Build history of the part. All positions in model axes, mm. Round coordinates to 2 decimals unless told otherwise and drop trailing zeros. Order: outer loops, then holes, each group sorted by start corner. A loop starts at its lowest first (then second) coordinate and runs counter-clockwise, first axis right, second up. Notation, with made-up numbers: (74, 58) -> (81, 58) arc R17 ccw to (81, 89) -> close; hole circle Ø3 at (14.5, 63). An arc over 180 degrees is marked (long way). Answer as a JSON object with one key per item and string values.
from build123d import *

# Parameters (mm, degrees)
SKETCH1_R           = 4.09575
SKETCH1_R_2         = 1.651
BOSS_EXTRUDE1_DEPTH = 6.35
SKETCH3_R           = 1.5875
CUT_EXTRUDE1_DEPTH  = 6.35
CUT_EXTRUDE2_DEPTH  = 6.35
SKETCH7_R           = 4.9784
CUT_EXTRUDE3_DEPTH  = 131.317526076
FILLET1_R           = 6.35
SKETCH8_W           = 50.8
SKETCH8_H           = 38.1
CUT_EXTRUDE4_DEPTH  = 50.8
CUT_EXTRUDE5_DEPTH  = 19.304
FILLET6_R           = 6.35
FILLET8_R           = 19.05
SKETCH10_R          = 1.5875
CUT_EXTRUDE6_DEPTH  = 6.35
SKETCH11_R          = 1.5875
CUT_EXTRUDE7_DEPTH  = 6.35
BOSS_EXTRUDE2_DEPTH = 6.35
FILLET9_R           = 24.13


with BuildPart() as part:
    # Sketch1 → Boss-Extrude1 (new body)
    with BuildSketch(Plane.XY):
        with BuildLine():
            Line((0, 0), (107.95, 0))
            Line((107.95, 0), (100.9362606, 26.175631792))
            Line((100.9362606, 26.175631792), (96.600438298, 42.357140917))
            ThreePointArc((96.600438298, 42.357140917), (108.063690957, 58.995863967), (92.935889192, 72.39))
            Line((92.935889192, 72.39), (0, 38.1))
            Line((0, 38.1), (0, 25.4))
            Line((0, 25.4), (-7.62, 25.4))
            Line((-7.62, 25.4), (-7.62, 12.7))
            Line((-7.62, 12.7), (0, 12.7))
            Line((0, 12.7), (0, 0))
        make_face()
        with Locations((92.935889192, 57.15)):
            Circle(SKETCH1_R, mode=Mode.SUBTRACT)
        with Locations((25.817011896, 25.817011896)):
            Circle(SKETCH1_R_2, mode=Mode.SUBTRACT)
        with Locations((25.817011896, 12.282988104)):
            Circle(SKETCH1_R_2, mode=Mode.SUBTRACT)
        with Locations((12.282988104, 12.282988104)):
            Circle(SKETCH1_R_2, mode=Mode.SUBTRACT)
        with Locations((12.282988104, 25.817011896)):
            Circle(SKETCH1_R_2, mode=Mode.SUBTRACT)
    extrude(amount=BOSS_EXTRUDE1_DEPTH)

    # Sketch3 → Cut-Extrude1 (cut)
    with BuildSketch(Plane.ZY):
        with Locations(Location((3.175, 31.75, 0), (0, 0, 270))):
            Circle(SKETCH3_R)
        with Locations(Location((3.175, 6.35, 0), (0, 0, 270))):
            Circle(SKETCH3_R)
    extrude(amount=-CUT_EXTRUDE1_DEPTH, mode=Mode.SUBTRACT)

    # Sketch6 → Cut-Extrude2 (cut)
    with BuildSketch(Plane.XY.offset(6.35)):
        with BuildLine():
            Line((50.8, 0), (76.2, 0))
            ThreePointArc((76.2, 0), (63.5, 12.7), (50.8, 0))
        make_face()
    extrude(amount=-CUT_EXTRUDE2_DEPTH, mode=Mode.SUBTRACT)

    # Sketch7 → Cut-Extrude3 (cut, through all)
    with BuildSketch(Plane.XY.offset(6.35)):
        with Locations((19.05, 19.05)):
            Circle(SKETCH7_R)
    extrude(amount=-CUT_EXTRUDE3_DEPTH, mode=Mode.SUBTRACT)

    # Fillet1
    fillet1_edges = [part.edges().sort_by_distance(p)[0] for p in [
        (96.600438298, 42.357140917, 3.175),
    ]]
    fillet(fillet1_edges, radius=FILLET1_R)

    # Sketch8 → Cut-Extrude4 (cut)
    with BuildSketch(Plane.XY.offset(6.35)):
        with Locations((25.4, 57.15)):
            Rectangle(SKETCH8_W, SKETCH8_H)
    extrude(amount=-CUT_EXTRUDE4_DEPTH, mode=Mode.SUBTRACT)

    # Sketch9 → Cut-Extrude5 (cut)
    with BuildSketch(Plane.XY.offset(6.35)):
        Polygon((50.8, 56.84337261), (50.8, 40.64), (57.15, 40.64), (57.15, 59.186294187), align=None)
    extrude(amount=-CUT_EXTRUDE5_DEPTH, mode=Mode.SUBTRACT)

    # Fillet6
    fillet6_edges = [part.edges().sort_by_distance(p)[0] for p in [
        (57.15, 40.64, 3.175),
    ]]
    fillet(fillet6_edges, radius=FILLET6_R - 0.0001)  # a hair under: the kernel refuses the full size

    # Fillet8
    fillet8_edges = [part.edges().sort_by_distance(p)[0] for p in [
        (50.8, 0, 3.175),
    ]]
    fillet(fillet8_edges, radius=FILLET8_R)

    # Sketch10 → Cut-Extrude6 (cut)
    with BuildSketch(Plane.XZ):
        with Locations(Location((97.79, 3.175, 0), (0, 0, 270))):
            Circle(SKETCH10_R)
        with Locations(Location((86.36, 3.175, 0), (0, 0, 270))):
            Circle(SKETCH10_R)
        with Locations(Location((31.75, 3.175, 0), (0, 0, 270))):
            Circle(SKETCH10_R)
        with Locations(Location((12.7, 3.175, 0), (0, 0, 270))):
            Circle(SKETCH10_R)
    extrude(amount=-CUT_EXTRUDE6_DEPTH, mode=Mode.SUBTRACT)

    # Sketch11 → Cut-Extrude7 (cut)
    with BuildSketch(Plane(origin=(0, 38.1, 0), x_dir=(1, 0, 0), z_dir=(0, 1, 0))):
        with Locations(Location((12.7, -2.922371253, 0), (0, 0, 270))):
            Circle(SKETCH11_R)
        with Locations(Location((25.4, -2.922371253, 0), (0, 0, 270))):
            Circle(SKETCH11_R)
        with Locations(Location((38.1, -2.922371253, 0), (0, 0, 270))):
            Circle(SKETCH11_R)
    extrude(amount=-CUT_EXTRUDE7_DEPTH, mode=Mode.SUBTRACT)

    # Sketch12 → Boss-Extrude2 (add)
    with BuildSketch(Plane.XY.offset(6.35)):
        with BuildLine():
            Line((50.8, 40.64), (85.027112904, 40.64))
            Line((85.027112904, 40.64), (92.935889192, 72.39))
            add(Edge.make_bspline(
                [(50.8, 40.64), (77.240642826, 53.266729026), (54.818289847, 129.190596971), (92.935889192, 72.39)],
                knots=[0, 0, 0, 0, 1, 1, 1, 1], degree=3))
        make_face()
    extrude(amount=-BOSS_EXTRUDE2_DEPTH)

    # Fillet9
    fillet9_edges = [part.edges().sort_by_distance(p)[0] for p in [
        (92.935889192, 72.39, 3.175),
    ]]
    fillet(fillet9_edges, radius=FILLET9_R)


solid = part.part
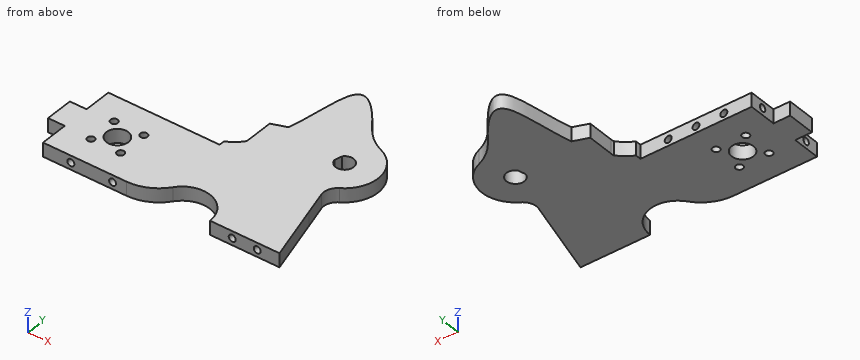
1) Cut at B-B, the plane y = 17.5. Give the cut face in (x, z).
Checked values:
{"outline": "(-7.62, 0) -> (14.32, 0) -> (14.32, 6.35) -> (-7.62, 6.35) -> close; (23.78, 0) -> (103.26, 0) -> (103.26, 6.35) -> (23.78, 6.35) -> close"}
2) Flat gauge pins, fed straight in: pin 1 Ø1 at (y, z) = (31.5, 2.5) entering from -X; pin 2 Ø3.5 at (x, z) = (86, 2.5) entering from -Y; pin 3 Ø3.5 at (x, z) = (12.7, 3.175) entering from +Y; pin 4 Ø1.9 at (y, z) = (7.5, 3) entering from -X. Where does each tip first touch, or does it go through?
Checked values:
{"pin 1": "stops at x = 6.35", "pin 2": "stops at y = 0", "pin 3": "stops at y = 38.1", "pin 4": "stops at x = 0"}
3) Cut at A-A, the plane x = 19.05. Give the cut face in (y, z), plus the area to 3 significant figures.
Checked values:
{"outline": "(0, 0) -> (14.07, 0) -> (14.07, 6.35) -> (0, 6.35) -> close; (24.03, 0) -> (38.1, 0) -> (38.1, 6.35) -> (24.03, 6.35) -> close", "area": "179 mm²"}
4) Probe L1, parallel to Y at x = 25.5, z = 3.5; L2, parallel to Y at x = 12.5, z = 2.75; L3, parallel to Z at x = 97.79, y = 2. List the from-to ranges inside material, lowest first. Write a range as from..to.
Checked values:
{"L1": "y = 0..10.66, 13.9..24.2, 27.44..31.75", "L2": "y = 6.35..10.65, 13.92..24.18, 27.45..31.75", "L3": "z = 0..1.59, 4.76..6.35"}
